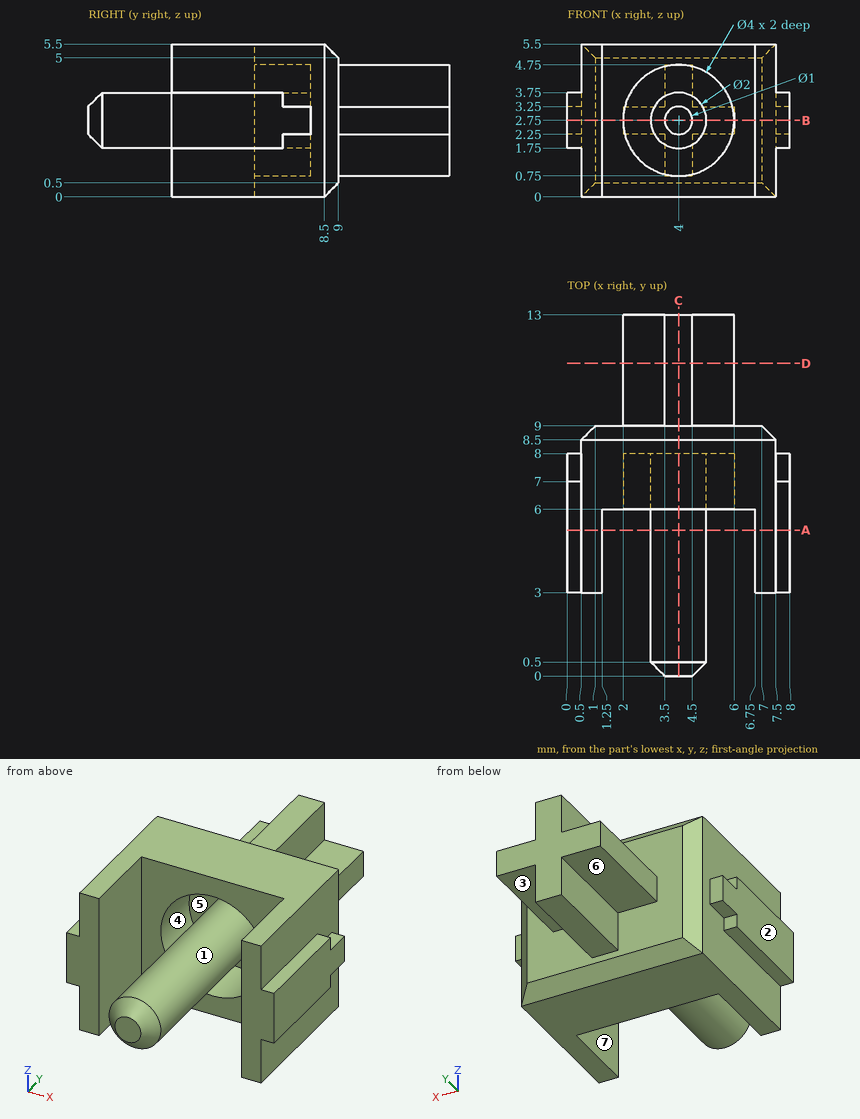
Job drawing, mm, ordinate dimensions from the low corner. One solid piece. A direction names the side the tool comes from. Round coordinates to 2 decimals unless told otherwise and drop trailing zeros. Order: outer loops, then holes, each group sorted by start corner. A loop starts at its lowest first (then second) coordinate and runs counter-clockwise, first axis right, second up. Notation, with made-up numbers: M 36,31 L 47,31 A20 ccw 47,66 Z; hole C 83,4 d3. An arc over 180 degrees is marked long. Write each question's results on one line, items separated by ' | '. Start each with the question number.
(1) Two-plate mould, pull along X, no slides. Class the marked faces 1, 2, 3 and 4: pulls with the +X half, pulls with the -X half, needs draft (parallel to the pull), parting line crosses it, or undercut.
(2) Drop flat-ended pins along their axis: pin 1 (0.5 mm diameter, centred on x = 4, y = 10.5, fed in from -Z); pin 2 (0.6 mm diameter, centred on x = 8, z = 3, fed in from +Y); pin 3 (2 mm diameter, centred on x = 7, z = 3, fed in from -Y). Give the stop position or say it passes through.
(3) Saw through at A-A, the plane y = 5.25. Give the cut face in (x, z), then the cut area to 3 significant figures.
(4) Saw through at C-C, the plane x = 4. Give the cut face in (y, z).
(5) Which spindle directions (+Z, -Z, +X, -X, +Y, -Y) get a long thin tool onto all of the face, cutting with end or side? Do the marked faces 5, 6 and 7. Say none if no direction does.
(6) Saw through at B-B, the plane z = 2.75. Give the cut face in (x, y), then the cut area to 3 significant figures.
(7) Probe probe 1 along X at (y, z) = (6.55, 2.75); probe 2 along X at (y, z) = (7.5, 1.15); probe 3 along Y at (x, z) = (5.5, 1.65). List the from-to ranges inside material, lowest first. Write a range as from..to.
(8) Saw through at D-D, the plane y = 11.25. Give the cut face in (x, z), then the cut area to 3 significant figures.
Established:
1) face 1: undercut | face 2: pulls with the -X half | face 3: needs draft | face 4: undercut
2) pin 1: stops at z = 0.75 | pin 2: stops at y = 8 | pin 3: stops at y = 3
3) outline: M 0,1.75 L 0.5,1.75 L 0.5,0 L 1.25,0 L 1.25,5.5 L 0.5,5.5 L 0.5,3.75 L 0,3.75 Z; C 4,2.75 d2; M 6.75,0 L 7.5,0 L 7.5,1.75 L 8,1.75 L 8,3.75 L 7.5,3.75 L 7.5,5.5 L 6.75,5.5 Z | area: 13.4 mm^2
4) outline: M 0,2.25 L 0.5,1.75 L 8,1.75 L 8,0.75 L 6,0.75 L 6,0 L 8.5,0 L 9,0.5 L 9,0.75 L 13,0.75 L 13,4.75 L 9,4.75 L 9,5 L 8.5,5.5 L 6,5.5 L 6,4.75 L 8,4.75 L 8,3.75 L 0.5,3.75 L 0,3.25 Z
5) face 5: -Y | face 6: -Z, -X, +Y | face 7: +Z, -Z, -Y
6) outline: M 0,3 L 1.25,3 L 1.25,6 L 2,6 L 2,8 L 3,8 L 3,0.5 L 3.5,0 L 4.5,0 L 5,0.5 L 5,8 L 6,8 L 6,6 L 6.75,6 L 6.75,3 L 8,3 L 8,8 L 7.5,8 L 7.5,8.5 L 7,9 L 6,9 L 6,13 L 2,13 L 2,9 L 1,9 L 0.5,8.5 L 0.5,8 L 0,8 Z | area: 54.0 mm^2
7) probe 1: x = 0..2, 3..5, 6..8 | probe 2: x = 0.5..2.8, 5.2..7.5 | probe 3: y = 8..9
8) outline: M 2,2.25 L 3.5,2.25 L 3.5,0.75 L 4.5,0.75 L 4.5,2.25 L 6,2.25 L 6,3.25 L 4.5,3.25 L 4.5,4.75 L 3.5,4.75 L 3.5,3.25 L 2,3.25 Z | area: 7.00 mm^2
